Check sheet for the drawn part. Datum: minimum x, y, z corner. Units: mm. A direction names the side the tool comes from. Coordinates: 2 decimals unless noted, no trailing zeros. Order: outer loops, then holes, each group sorted by start corner. A loop starts at its lowest first (then second) coordinate and runs counter-clockwise, first axis right, second up.
1. Draft check along X on the marked faces 1 and 2. Enter one of: released by +X, released by -X, zero draft, split by the parting line, or undercut.
2. Cross-section at D-D (y = 74.5). Enter the section's corners in (x, z), then the cut area to 3 significant figures.
3. Thickness scan on line 1 (Z direction, x = 45.5, y = 45); line 2 (Y direction, x = 89, z = 17); line 3 (Y direction, x = 85, z = 80). Record the ranges inside material, lowest first.
4. Set-up check for the marked faces 3 and 4: record each of +Z, -Z, +X, -X, +Y, -Y from which the full face is reachable in a straight line by a thin tool's end or side.
5. Gauge pin test, flat ends, axial feed: pin 1 Ø8 at (y, z) = (44.5, 45) entering from +X; pin 2 Ø5 at (y, z) = (22, 65) entering from -X; pin 3 Ø1 at (x, y) = (69, 105.5) entering from +Z; pin 4 Ø5 at (x, y) = (99.5, 61) entering from -Z. Record the tip position at first contact, or that the pin passes through.
6. Cross-section at C-C (y = 19). Enter the section's corners in (x, z).
7. Cross-section at A-A (x = 63.5). Enter the section's corners in (y, z) (3 decimals), then the cut area to 3 significant figures.
8. Cross-section at B-B (z = 63.5). Enter the section's corners in (x, y) (3 decimals).
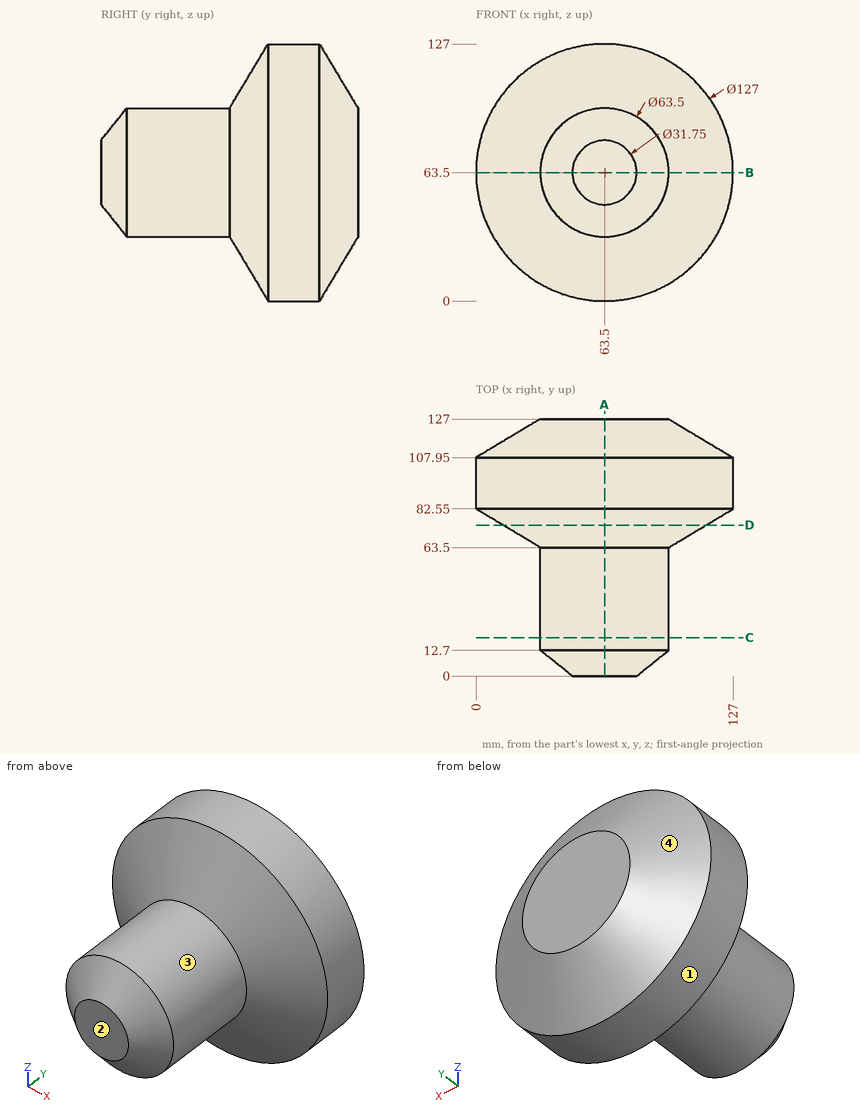
Data:
1. face 1: split by the parting line
1. face 2: zero draft
2. outline: circle Ø100.17 at (63.5, 63.5)
2. area: 7,880 mm2
3. line 1: z = 37.35 to 89.65
3. line 2: y = 76.27 to 114.23
3. line 3: y = 8.98 to 127
4. face 3: -Y
4. face 4: +Y
5. pin 1: stops at x = 91.75
5. pin 2: stops at x = 31.75
5. pin 3: stops at z = 126.8
5. pin 4: passes through
6. outline: circle Ø63.5 at (63.5, 63.5)
7. outline: (0, 47.625) - (12.7, 31.75) - (63.5, 31.75) - (82.55, 0) - (107.95, 0) - (127, 31.75) - (127, 95.25) - (107.95, 127) - (82.55, 127) - (63.5, 95.25) - (12.7, 95.25) - (0, 79.375) - close
7. area: 10,700 mm2
8. outline: (0, 82.55) - (31.75, 63.5) - (31.75, 12.7) - (47.625, 0) - (79.375, 0) - (95.25, 12.7) - (95.25, 63.5) - (127, 82.55) - (127, 107.95) - (95.25, 127) - (31.75, 127) - (0, 107.95) - close
